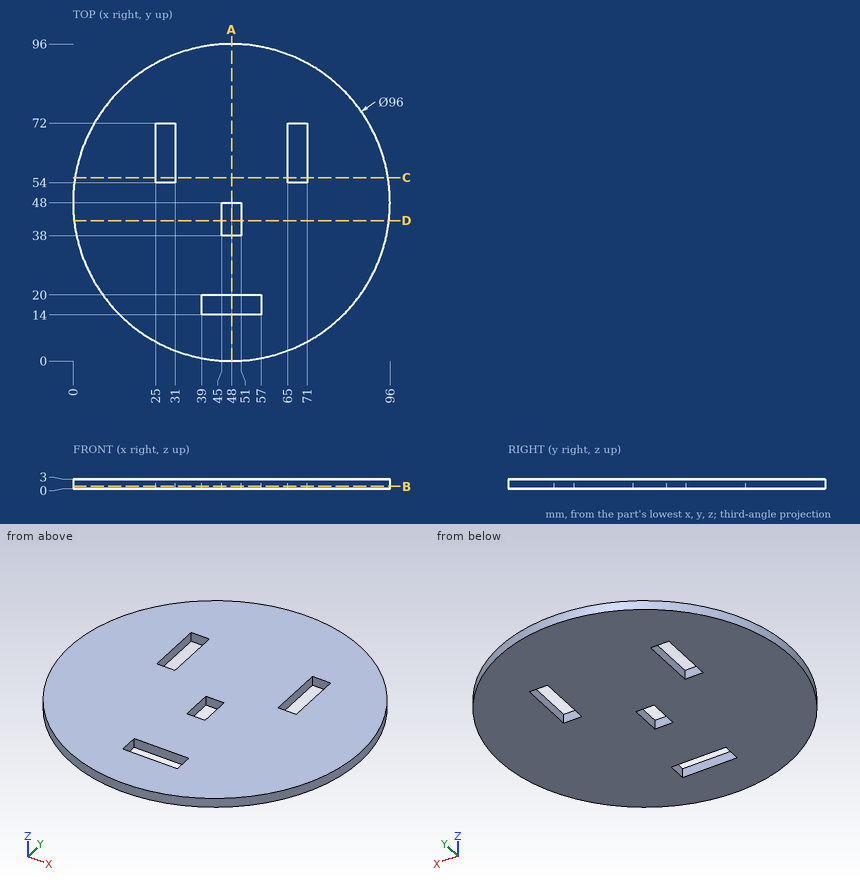
Study the drawing (mm; zero at the part's minimum x, y, z) and answer. Give positions to 0.01 mm unless a question says otherwise; leave off trailing zeros. Order: outer loops, then holes, each group sorted by start corner. A loop starts at its lowest first (then second) coordinate and runs counter-clockwise, first axis right, second up. Notation, with made-up numbers: M -2,15 L 45,15 A24 cw 45,50 Z; hole C -17,45 d9. An arc over 180 degrees is marked long. Put each result on its own line as item: value. Start each with the question number.
Item 1: The part is cut by section A-A, the plane x = 48. Determine the outline of the cut face in (y, z), and give its area (3 significant figures).
Item 2: The part is cut by section B-B, the plane z = 0.8. Determine the outline of the cut face in (x, y), and give its area (3 significant figures).
Item 3: The part is cut by section C-C, the plane y = 55.5. Determine the outline of the cut face in (x, z).
Item 4: The part is cut by section D-D, the plane y = 42.5. Determine the outline of the cut face in (x, z).
Item 5: Flat-ended cylindrical pins translate along their axes: P1, Ø1, axis at x = 34, z = 2, coming from the +Y side; P2, Ø0.9, axis at y = 58.5, z = 1.5, coming from the -X side; P3, Ø0.9, axis at y = 65.5, z = 2, coming from the -X side. Find the tip coordinate at first contact, or state that the pin passes through.
Item 6: Find the intervals of material crossed by line 1 along X through (y, z) = (58.5, 1.65); line 2 along X through (y, z) = (58, 0.3); line 3 along Y through (x, z) = (69, 1.85), in increasing order.
Answer key:
1. outline: M 0,0 L 14,0 L 14,3 L 0,3 Z; M 20,0 L 38,0 L 38,3 L 20,3 Z; M 48,0 L 96,0 L 96,3 L 48,3 Z
1. area: 240 mm²
2. outline: C 48,48 d96; hole M 25,54 L 31,54 L 31,72 L 25,72 Z; hole M 39,14 L 57,14 L 57,20 L 39,20 Z; hole M 45,38 L 51,38 L 51,48 L 45,48 Z; hole M 65,54 L 71,54 L 71,72 L 65,72 Z
2. area: 6,850 mm²
3. outline: M 0.59,0 L 25,0 L 25,3 L 0.59,3 Z; M 31,0 L 65,0 L 65,3 L 31,3 Z; M 71,0 L 95.41,0 L 95.41,3 L 71,3 Z
4. outline: M 0.32,0 L 45,0 L 45,3 L 0.32,3 Z; M 51,0 L 95.68,0 L 95.68,3 L 51,3 Z
5. P1: stops at y = 94.06
5. P2: stops at x = 1.06
5. P3: stops at x = 3.13
6. line 1: x = 1.16 to 25, 31 to 65, 71 to 94.84
6. line 2: x = 1.05 to 25, 31 to 65, 71 to 94.95
6. line 3: y = 4.84 to 54, 72 to 91.16
